For this review, take the finished solid that the model builds, in its own axes (mm). Coordinates: 2 decimals unless noted, no trailing zeros. Order: outer loops, then holes, each group sorted by start corner. A loop starts at its lowest first (then second) coordinate and runs counter-clockwise, first axis right, second up. Notation, with made-up numbers: (-18, -8) -> (-6, -8) arc R29 cw to (-6, 19) -> close; hole circle Ø9 at (77.5, 85.25). An arc over 180 degrees is marked (long way). Answer as a JSON object with one key per item and string values. Group by question number.
1) Add section A-A, the plane y = 642.5. Write out the cut boundary in (x, z) (3 decimals).
2) Draft analysis for pull direction Z (two halves, no side actions). For faces 1 (the flat face through (269, 25.4, -214)), 2 (the flat face through (288.925, 714, -216)), 3 (the flat face through (279, 714, -241.3)), 4 (the flat face through (269.875, 714, -216)), state which applies: +Z half, -Z half, draft (parallel to the pull), parting line (faces both ways), or undercut.
3) Add section B-B, the plane z = -204.5. Write out the cut boundary in (x, y) (3 decimals).
4) Wall thickness on L1, parallel to Y at x = 279.4, z = -239.6 (3 decimals); L2, parallel to X at y = 933.5, z = -217.5 (3 decimals); L3, parallel to X at y = 1409.7, z = -239.8 (3 decimals): over which ranges is each line inside the solid? List them lowest first.
from build123d import *

# Parameters (mm, degrees)
SKETCH1_W               = 25.4
SKETCH1_H               = 50.8
SKETCH1_W_2             = 19.05
SKETCH1_H_2             = 44.45
BOSS_EXTRUDE1_DEPTH     = 1397
SKETCH2_R               = 3.2639
CUT_EXTRUDE1_DEPTH      = 1472.995197003
CUT_EXTRUDE2_DEPTH      = 1472.995197003
CUT_EXTRUDE2_DEPTH_BACK = 1472.995197003
SKETCH3_R               = 3.175


with BuildPart() as part:
    # Sketch1 → Boss-Extrude1 (new body)
    with BuildSketch(Plane(origin=(0, 25.4, 0), x_dir=(1, 0, 0), z_dir=(0, 1, 0))):
        with Locations((279.4, 215.9)):
            Rectangle(SKETCH1_W, SKETCH1_H)
        with Locations((279.4, 215.9)):
            Rectangle(SKETCH1_W_2, SKETCH1_H_2, mode=Mode.SUBTRACT)
    extrude(amount=BOSS_EXTRUDE1_DEPTH)

    # Sketch2 → Cut-Extrude1 (cut, through all)
    with BuildSketch(Plane.XY):
        with Locations((279.4, 1314.45)):
            Circle(SKETCH2_R)
        with Locations((279.4, 1352.55)):
            Circle(SKETCH2_R)
    extrude(amount=-CUT_EXTRUDE1_DEPTH, mode=Mode.SUBTRACT)

    # Sketch3 → Cut-Extrude2 (cut, two sides: drawn at the far end of the back side and taken through both)
    with BuildSketch(Plane.XY.offset(-CUT_EXTRUDE2_DEPTH_BACK)):
        with Locations((279.4, 1384.3)):
            Circle(SKETCH3_R)
        with Locations((279.4, 1409.7)):
            Circle(SKETCH3_R)
    extrude(amount=CUT_EXTRUDE2_DEPTH + CUT_EXTRUDE2_DEPTH_BACK, mode=Mode.SUBTRACT)


solid = part.part
Output values:
{
 "1": {"outline": "(266.7, -241.3) -> (292.1, -241.3) -> (292.1, -190.5) -> (266.7, -190.5) -> close; hole (269.875, -238.125) -> (288.925, -238.125) -> (288.925, -193.675) -> (269.875, -193.675) -> close"},
 "2": {"face 1": "draft", "face 2": "undercut", "face 3": "-Z half", "face 4": "undercut"},
 "3": {"outline": "(266.7, 25.4) -> (269.875, 25.4) -> (269.875, 1422.4) -> (266.7, 1422.4) -> close; (288.925, 25.4) -> (292.1, 25.4) -> (292.1, 1422.4) -> (288.925, 1422.4) -> close"},
 "4": {"L1": "y = 25.4 to 1311.186, 1317.714 to 1349.286, 1355.814 to 1381.125, 1387.475 to 1406.525, 1412.875 to 1422.4", "L2": "x = 266.7 to 269.875, 288.925 to 292.1", "L3": "x = 266.7 to 276.225, 282.575 to 292.1"}
}
